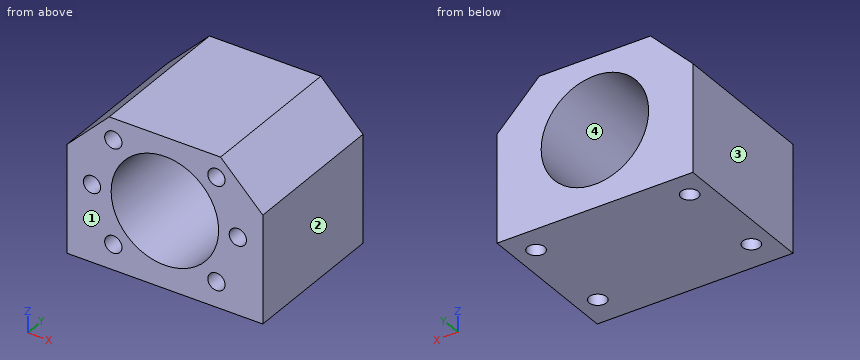
```python
from build123d import *

# Parameters (mm, degrees)
F0_R     = 2.25
F0_R_2   = 14
F2_DEPTH = 39
F3_DEPTH = 29
F1_R     = 2.25
F4_DEPTH = 25


with BuildPart() as f2:
    # F0 (on Front) → F2 (new body)
    with BuildSketch(Plane.XZ):
        Polygon((-25.5, -14), (25.5, -14), (25.5, 14), (14.5, 25), (-14.5, 25), (-25.5, 14), align=None)
        with Locations((-13.435029, -7.435029)):
            Circle(F0_R, mode=Mode.SUBTRACT)
        with Locations((13.435029, -7.435029)):
            Circle(F0_R, mode=Mode.SUBTRACT)
        with Locations((-19, 6)):
            Circle(F0_R, mode=Mode.SUBTRACT)
        with Locations((-13.435029, 19.435029)):
            Circle(F0_R, mode=Mode.SUBTRACT)
        with Locations((0, 6)):
            Circle(F0_R_2, mode=Mode.SUBTRACT)
        with Locations((19, 6)):
            Circle(F0_R, mode=Mode.SUBTRACT)
        with Locations((13.435029, 19.435029)):
            Circle(F0_R, mode=Mode.SUBTRACT)
    extrude(amount=F2_DEPTH)

    # F0 (on Front) → F3 (join)
    with BuildSketch(Plane.XZ):
        with Locations((19, 6)):
            Circle(F0_R)
        with Locations((13.435029, 19.435029)):
            Circle(F0_R)
        with Locations((13.435029, -7.435029)):
            Circle(F0_R)
        with Locations((-13.435029, -7.435029)):
            Circle(F0_R)
        with Locations((-19, 6)):
            Circle(F0_R)
        with Locations((-13.435029, 19.435029)):
            Circle(F0_R)
    extrude(amount=F3_DEPTH)

    # F1 (on face) → F4 (cut)
    with BuildSketch(Plane(origin=(0, 0, -14), x_dir=(1, 0, 0), z_dir=(0, 0, -1))):
        with Locations((-20, 7)):
            Circle(F1_R)
        with Locations((-20, 31)):
            Circle(F1_R)
        with Locations((20, 31)):
            Circle(F1_R)
        with Locations((20, 7)):
            Circle(F1_R)
    extrude(amount=-F4_DEPTH, mode=Mode.SUBTRACT)


solid = f2.part
```
The model under review builds one solid part; all positions refer to its coordinate system, in mm. Face numbers are marked on the shaded views. Round coordinates to 2 decimals unless told otherwise and drop trailing zeros. Loops run counter-clockwise (first coordinate to the right, second up) from the corner with the lowest first, then second, coordinate; pieces in that order, holes last.
Item 1: Clearance check with flat-ended pins moving along their axes: pin 1 Ø2.5 at (x, z) = (13.44, 19.44) entering from -Y; pin 2 Ø4 at (x, y) = (20, -31) entering from -Z; pin 3 Ø6 at (x, y) = (20, -7) entering from +Z. State where each tip first meets the part, or that it passes through.
Determined:
pin 1: stops at y = -29
pin 2: stops at z = 11
pin 3: stops at z = 22.5
Item 2: Mouldability with a two-part tool opening along X and no side actions: class the marked faces 1, 2, 3 and 4 as released by +X, released by -X, zero draft, split by the parting line, or undercut.
Determined:
face 1: zero draft
face 2: released by +X
face 3: released by -X
face 4: undercut
Item 3: Take a section at C-C (y = -7). Write out the cut boundary in (x, z), then the cut area to 3 significant figures.
Determined:
outline: (-25.5, -14) - (-22.25, -14) - (-22.25, 11) - (-17.75, 11) - (-17.75, -14) - (17.75, -14) - (17.75, 11) - (22.25, 11) - (22.25, -14) - (25.5, -14) - (25.5, 14) - (14.5, 25) - (-14.5, 25) - (-25.5, 14) - close; hole circle Ø28 at (0, 6)
area: 1,030 mm2
Item 4: Take a section at A-A (z = 6). Write out the cut boundary in (x, y).
Determined:
outline: (-25.5, -39) - (-21.25, -39) - (-21.25, -32.87) arc R2.25 cw to (-21.25, -29.13) - (-21.25, -29) - (-21.03, -29) arc R2.25 cw to (-18.97, -29) - (-16.75, -29) - (-16.75, -39) - (-14, -39) - (-14, 0) - (-25.5, 0) - close; (14, -39) - (16.75, -39) - (16.75, -29) - (18.97, -29) arc R2.25 cw to (21.03, -29) - (21.25, -29) - (21.25, -29.13) arc R2.25 cw to (21.25, -32.87) - (21.25, -39) - (25.5, -39) - (25.5, 0) - (14, 0) - close; hole circle Ø4.5 at (-20, -7); hole circle Ø4.5 at (20, -7)
Item 5: For line 1 (Y direction, x = -20, z = -4); line 2 (Y direction, x = -21, z = -5); line 3 (Z direction, x = 0.5, y = -23), list the stretches that pass through material, from the lowest coordinate up.
Determined:
line 1: y = -39 to -33.25, -28.75 to -9.25, -4.75 to 0
line 2: y = -39 to -33.02, -28.98 to -9.02, -4.98 to 0
line 3: z = -14 to -7.99, 19.99 to 25
Item 6: Take a section at D-D (z = 12.5). Write out the cut boundary in (x, y).
Determined:
outline: (-25.5, -39) - (-12.4, -39) - (-12.4, 0) - (-25.5, 0) - close; (12.4, -39) - (25.5, -39) - (25.5, 0) - (12.4, 0) - close
Item 7: Take a section at B-B (x = 0). Write out the cut boundary in (y, z), then the cut area to 3 significant figures.
Determined:
outline: (-39, -14) - (0, -14) - (0, -8) - (-39, -8) - close; (-39, 20) - (0, 20) - (0, 25) - (-39, 25) - close
area: 429 mm2
